Read the model definition and answer for the solid it produces. Units are mm, in the model's axes. Give positions to 0.01 mm unless a question says otherwise; leave off trailing zeros. Write each loop counter-clockwise with the first axis right and the second up, starting at its lowest first coordinate (ties: lowest second). Pieces come first, ordered by that corner, then holes. Notation, with made-up numbers: (49, 18.5) - (79, 18.5) arc R6 cw to (79, 28.5) - close; hole circle Ø1 at (-34, -19). An arc over 180 degrees is marked (long way). Answer as CSV lines item,"result".
```python
from build123d import *

# Parameters (mm, degrees)
SKETCH1_R           = 1.5
SKETCH1_R_2         = 11.5
BOSS_EXTRUDE1_DEPTH = 4
FILLET1_R           = 3


with BuildPart() as part:
    # Sketch1 → Boss-Extrude1 (new body)
    with BuildSketch(Plane.XY):
        with BuildLine():
            Line((-20.616075737, 20.616075737), (-63.042482608, -21.810331134))
            ThreePointArc((-63.042482608, -21.810331134), (-64.214055483, -24.638758259), (-63.042482608, -27.467185384))
            add(Edge.make_bspline(
                [(-2.828427125, -32.7468701), (-22.744659396, -52.590484488), (-57.268164388, -33.201805253), (-63.042482608, -27.467185384)],
                knots=[0, 0, 0, 0, 1, 1, 1, 1], degree=3))
            ThreePointArc((-2.828427125, -32.7468701), (0, -31.575297224), (2.828427125, -32.7468701))
            ThreePointArc((2.828427125, -32.7468701), (5.656854249, -33.918442975), (8.485281374, -32.7468701))
            Line((8.485281374, -32.7468701), (32.7468701, -8.485281374))
            ThreePointArc((32.7468701, -8.485281374), (33.918442975, -5.656854249), (32.7468701, -2.828427125))
            Line((32.7468701, -2.828427125), (0, 29.918442975))
            Line((0, 29.918442975), (-9.302367238, 20.616075737))
            ThreePointArc((-9.302367238, 20.616075737), (-12.130794363, 19.444502862), (-14.959221487, 20.616075737))
            ThreePointArc((-14.959221487, 20.616075737), (-17.787648612, 21.787648612), (-20.616075737, 20.616075737))
        make_face()
        with Locations((29.918442975, -5.656854249)):
            Circle(SKETCH1_R, mode=Mode.SUBTRACT)
        with Locations((-21.920310217, 0)):
            Circle(SKETCH1_R, mode=Mode.SUBTRACT)
        with Locations((0, 21.920310217)):
            Circle(SKETCH1_R, mode=Mode.SUBTRACT)
        with Locations((21.920310217, 0)):
            Circle(SKETCH1_R, mode=Mode.SUBTRACT)
        Circle(SKETCH1_R_2, mode=Mode.SUBTRACT)
        with Locations((0, -21.920310217)):
            Circle(SKETCH1_R, mode=Mode.SUBTRACT)
        with Locations((5.656854249, -29.918442975)):
            Circle(SKETCH1_R, mode=Mode.SUBTRACT)
        with Locations((-17.787648612, 17.787648612)):
            Circle(SKETCH1_R, mode=Mode.SUBTRACT)
        with Locations((-60.214055483, -24.638758259)):
            Circle(SKETCH1_R, mode=Mode.SUBTRACT)
    extrude(amount=BOSS_EXTRUDE1_DEPTH)

    # Fillet1
    fillet1_edges = [part.edges().sort_by_distance(p)[0] for p in [
        (0, 29.918442975, 2),
    ]]
    fillet(fillet1_edges, radius=FILLET1_R)


solid = part.part
```
(1) Find the intervals of material crossed by L1, parallel to Y at x = 0, z = 2.35; L2, parallel to Y at x = 0.5, z = 2.4; L3, parallel to X at y = -33.5, z = 3.25, in increasing order.
Worked out:
L1,"y = -31.58 to -23.42, -20.42 to -11.5, 11.5 to 20.42, 23.42 to 28.68"
L2,"y = -31.61 to -23.33, -20.51 to -11.49, 11.49 to 20.51, 23.33 to 28.63"
L3,"x = -54 to -3.61, 3.88 to 7.44"
(2) A cutting plane is placed at C-C (y = -10). Write down the section's boundary in (x, z), and give its area (3 significant figures).
Worked out:
outline,"(-51.23, 0) - (-5.68, 0) - (-5.68, 4) - (-51.23, 4) - close; (5.68, 0) - (31.23, 0) - (31.23, 4) - (5.68, 4) - close"
area,"284 mm^2"
(3) Each of these flat-tipped pins is pushed along its axis until it touches: P1, Ø2, axis at y = -22, z = 1, coming from the +X side; P2, Ø2.5, axis at x = 5.66, y = -29.92, coming from the -Z side; P3, Ø1, axis at y = 12, z = 2, coming from the -X side. Where does it stop, or does it pass through?
Worked out:
P1,"stops at x = 20.23"
P2,"passes through"
P3,"stops at x = -29.73"
(4) A cutting plane is placed at D-D (z = 3.05). Count the separate pieces of the cut face and the enclosed holes in it, and give its area (3 significant figures).
Worked out:
separate pieces,"1"
enclosed holes,"9"
area,"3,560 mm^2"
(5) The mould has two halves that part along Y. Classify faces 1 (the cylindrical face through (-64.214, -24.595, 1.972)), 2 (the cylindrical face through (6.46, -28.65, 1.97)), 3 (the flat face through (-16, -11, 4)): +Y half, -Y half, draft (parallel to the pull), parting line (faces both ways), or undercut.
Worked out:
face 1,"parting line"
face 2,"undercut"
face 3,"draft"
(6) A cutting plane is placed at B-B (y = 0). Write down the section's boundary in (x, z), and give its area (3 significant figures).
Worked out:
outline,"(-41.23, 0) - (-23.42, 0) - (-23.42, 4) - (-41.23, 4) - close; (-20.42, 0) - (-11.5, 0) - (-11.5, 4) - (-20.42, 4) - close; (11.5, 0) - (20.42, 0) - (20.42, 4) - (11.5, 4) - close; (23.42, 0) - (29.92, 0) - (29.92, 4) - (23.42, 4) - close"
area,"169 mm^2"
(7) A cutting plane is placed at A-A (x = 0). Write down the section's boundary in (y, z), and give its area (3 significant figures).
Worked out:
outline,"(-31.58, 0) - (-23.42, 0) - (-23.42, 4) - (-31.58, 4) - close; (-20.42, 0) - (-11.5, 0) - (-11.5, 4) - (-20.42, 4) - close; (11.5, 0) - (20.42, 0) - (20.42, 4) - (11.5, 4) - close; (23.42, 0) - (28.68, 0) - (28.68, 4) - (23.42, 4) - close"
area,"125 mm^2"
